The listing builds one solid part. Answer for the finished solid, in the listing's coordinates (mm). Round coordinates to 2 decimals unless told otherwise and drop trailing zeros. Order: outer loops, then holes, each group sorted by start corner. A loop starts at its lowest first (then second) coordinate and runs counter-clockwise, first axis right, second up. Notation, with made-up numbers: (56.25, 14.5) - (80.25, 14.5) arc R20 cw to (80.25, 43.5) - close; hole circle Ø7 at (-19.5, 29.5). An arc over 180 degrees is marked (long way). Use CSV: the item, a comma, the result in double quotes. Start each with the question number.
Item 1: Find section B-B, the plane y = -3.25. Count the separate pieces of the cut face and the enclosed holes in it, plus the area to 3 significant figures.
Item 2: Straight lines are drawn through the part: line 1 along Z through (x, y) = (16, -4.75); line 2 along X through (y, z) = (-6.25, -65); line 3 along Z through (x, y) = (-15.5, -6.4). For each, find the intervals that lie inside material, in ascending order. Write a range as [from, to].
Item 3: Find section A-A, the plane z = -16.5. Give the vertices of the cut face in (x, y), plus the area to 3 significant figures.
Item 4: Find section C-C, the plane z = -91.5. Give the vertices of the cut face in (x, y).
Item 5: Flat-ended cylindrical pins translate along their axes: P1, Ø3.5, axis at x = -13, z = -15, coming from the -Y side; P2, Ø4, axis at x = 15.5, z = 16.5, coming from the -Y side; P3, Ø2, axis at y = -2, z = -48.5, coming from the -X side; P4, Ø3, axis at x = 24.5, y = -2.5, coming from the -Z side. Find the tip coordinate at first contact, or state that the pin passes through.
```python
from build123d import *

# Parameters (mm, degrees)
F0_W      = 51
F0_H      = 60
F1_DEPTH  = 7
F2_R      = 3.5
F3_DEPTH  = 25
F4_R      = 5.5
F5_DEPTH  = 1
F6_W      = 43
F6_H      = 80
F7_DEPTH  = 7
F9_R      = 3.5
F10_DEPTH = 25
F11_R     = 5.5
F12_DEPTH = 1
F13_W     = 43
F13_H     = 8
F14_DEPTH = 25


with BuildPart() as f1:
    # F0 (on Front) → F1 (new body)
    with BuildSketch(Plane.XZ):
        Rectangle(F0_W, F0_H)
    extrude(amount=F1_DEPTH)

    # F2 (on face) → F3 (cut)
    with BuildSketch(Plane.XZ.offset(7)):
        with Locations((-15.5, 16.5)):
            Circle(F2_R)
        with Locations((-15.5, -16.5)):
            Circle(F2_R)
        with Locations((15.5, 16.5)):
            Circle(F2_R)
        with Locations((15.5, -16.5)):
            Circle(F2_R)
    extrude(amount=-F3_DEPTH, mode=Mode.SUBTRACT)

    # F4 (on face) → F5 (cut)
    with BuildSketch(Plane.XZ.offset(7)):
        with Locations((-15.5, 16.5)):
            Circle(F4_R)
        with Locations((-15.5, -16.5)):
            Circle(F4_R)
        with Locations((15.5, -16.5)):
            Circle(F4_R)
        with Locations((15.5, 16.5)):
            Circle(F4_R)
    extrude(amount=-F5_DEPTH, mode=Mode.SUBTRACT)


with BuildPart() as f7:
    # F6 (on face) → F7 (new body)
    with BuildSketch(Plane.XZ.offset(7)):
        with Locations((0, -70)):
            Rectangle(F6_W, F6_H)
    extrude(amount=-F7_DEPTH)


with BuildPart() as f1_1:
    add(f1.part)

    # F8: union F7
    add(f7.part)

    # F9 (on face) → F10 (cut)
    with BuildSketch(Plane.XZ.offset(7)):
        with Locations((-13, -61.5)):
            Circle(F9_R)
        with Locations((13, -61.5)):
            Circle(F9_R)
        with Locations((-13, -91.5)):
            Circle(F9_R)
        with Locations((13, -91.5)):
            Circle(F9_R)
    extrude(amount=-F10_DEPTH, mode=Mode.SUBTRACT)

    # F11 (on face) → F12 (cut)
    with BuildSketch(Plane.XZ.offset(7)):
        with Locations((-13, -61.5)):
            Circle(F11_R)
        with Locations((13, -61.5)):
            Circle(F11_R)
        with Locations((-13, -91.5)):
            Circle(F11_R)
        with Locations((13, -91.5)):
            Circle(F11_R)
    extrude(amount=-F12_DEPTH, mode=Mode.SUBTRACT)

    # F13 (on face) → F14 (cut)
    with BuildSketch(Plane.XZ.offset(7)):
        with Locations((0, -106)):
            Rectangle(F13_W, F13_H)
    extrude(amount=-F14_DEPTH, mode=Mode.SUBTRACT)


solid = f1_1.part
```
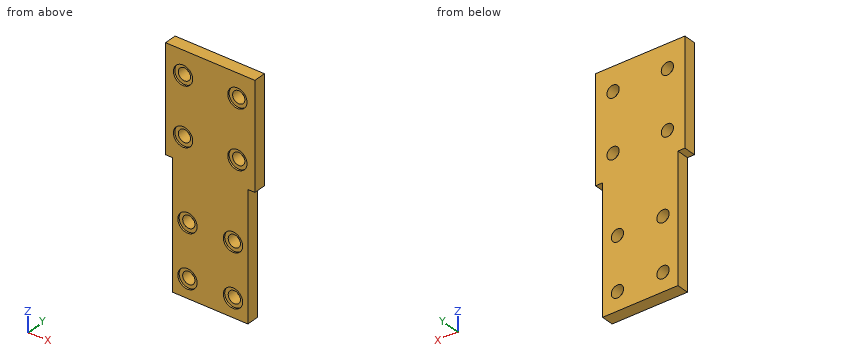
Worked out:
1,separate pieces,"1"
1,enclosed holes,"8"
1,area,"5,850 mm²"
2,line 1,"z = [-102, -93.3], [-89.7, -63.3], [-59.7, -19.96], [-13.04, 13.04], [19.96, 30]"
2,line 2,"x = [-21.5, -17.24], [-8.76, 8.76], [17.24, 21.5]"
2,line 3,"z = [-102, -96.4], [-86.6, -66.4], [-56.6, -22], [-11, 11], [22, 30]"
3,outline,"(-25.5, -7) - (-21, -7) - (-21, -6) - (-19, -6) - (-19, 0) - (-25.5, 0) - close; (-12, -6) - (-10, -6) - (-10, -7) - (10, -7) - (10, -6) - (12, -6) - (12, 0) - (-12, 0) - close; (19, -6) - (21, -6) - (21, -7) - (25.5, -7) - (25.5, 0) - (19, 0) - close"
3,area,"251 mm²"
4,outline,"(-21.5, -7) - (-18.5, -7) - (-18.5, -6) - (-16.5, -6) - (-16.5, 0) - (-21.5, 0) - close; (-9.5, -6) - (-7.5, -6) - (-7.5, -7) - (7.5, -7) - (7.5, -6) - (9.5, -6) - (9.5, 0) - (-9.5, 0) - close; (16.5, -6) - (18.5, -6) - (18.5, -7) - (21.5, -7) - (21.5, 0) - (16.5, 0) - close"
5,P1,"stops at y = -6"
5,P2,"passes through"
5,P3,"stops at x = -21.5"
5,P4,"stops at z = -30"
